Input: part model. Units: mm. Frame: model coordinates. Face numbers are marked on the shaded views. A direction names the side the tool comes from. Coordinates: 2 decimals unless noted, no trailing zeros. Order: outer loops, then holes, each group sorted by start corner. A loop starts at its lowest first (then second) coordinate and runs counter-clockwise, first axis right, second up.
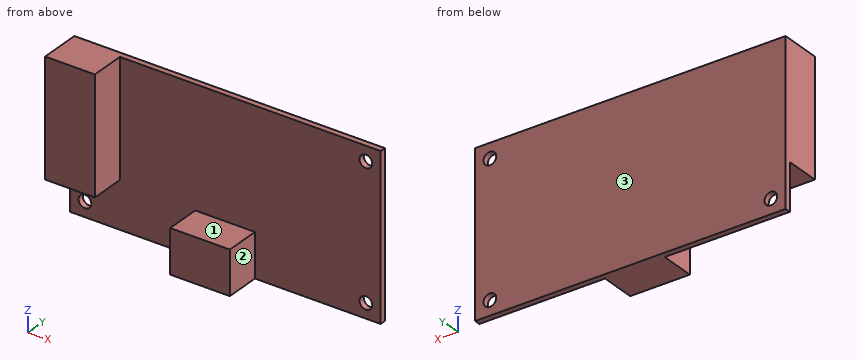
from build123d import *

# Parameters (mm, degrees)
SKETCH1_W           = 53.34
SKETCH1_H           = 27.94
SKETCH1_R           = 1.0922
BOSS_EXTRUDE1_DEPTH = 1
SKETCH2_W           = 8.533603159
SKETCH2_H           = 19.883520928
SKETCH2_W_2         = 10.243705623
SKETCH2_H_2         = 7.528700328
BOSS_EXTRUDE2_DEPTH = 7


with BuildPart() as part:
    # Sketch1 → Boss-Extrude1 (new body)
    with BuildSketch(Plane(origin=(0, 0, 0), x_dir=(1, 0, 0), z_dir=(0, 1, 0))):
        Rectangle(SKETCH1_W, SKETCH1_H)
        with Locations(Location((-24.13, 11.43, 0), (0, 0, 270))):
            Circle(SKETCH1_R, mode=Mode.SUBTRACT)
        with Locations(Location((24.13, 11.43, 0), (0, 0, 270))):
            Circle(SKETCH1_R, mode=Mode.SUBTRACT)
        with Locations(Location((24.13, -11.43, 0), (0, 0, 270))):
            Circle(SKETCH1_R, mode=Mode.SUBTRACT)
    extrude(amount=BOSS_EXTRUDE1_DEPTH)

    # Sketch2 → Boss-Extrude2 (add)
    with BuildSketch(Plane(origin=(0, 1, 0), x_dir=(1, 0, 0), z_dir=(0, 1, 0))):
        with Locations((-22.403198421, -4.028239536)):
            Rectangle(SKETCH2_W, SKETCH2_H)
        with Locations((-0.059974857, 10.205649836)):
            Rectangle(SKETCH2_W_2, SKETCH2_H_2)
    extrude(amount=-BOSS_EXTRUDE2_DEPTH)


solid = part.part
Item 1: Ray query, probe 1 along X at (y, z) = (0.5, -11.43); probe 2 along X at (y, z) = (0.2, 11.43); probe 3 along Z at (x, y) = (5, -0.75). Return the intervals inside material, ascending.
Response values:
probe 1: x = -26.67 to -25.22, -23.04 to 23.04, 25.22 to 26.67
probe 2: x = -26.67 to 23.04, 25.22 to 26.67
probe 3: z = -13.97 to -6.44
Item 2: Cut plane C-C on x = -24.13. Return loops of the section in (y, z), then the cut area to 3 significant figures.
Response values:
outline: (-6, -5.91) - (0, -5.91) - (0, -10.34) - (1, -10.34) - (1, 13.97) - (-6, 13.97) - close; (0, -13.97) - (1, -13.97) - (1, -12.52) - (0, -12.52) - close
area: 145 mm2
Item 3: Cut plane B-B on z = 11.43. Return loops of the section in (x, y).
Response values:
outline: (-26.67, -6) - (-18.14, -6) - (-18.14, 0) - (23.04, 0) - (23.04, 1) - (-26.67, 1) - close; (25.22, 0) - (26.67, 0) - (26.67, 1) - (25.22, 1) - close
Item 4: Cut plane D-D on z = -11.43. Return loops of the section in (x, y), then the cut area to 3 significant figures.
Response values:
outline: (-26.67, 0) - (-25.22, 0) - (-25.22, 1) - (-26.67, 1) - close; (-23.04, 0) - (-5.18, 0) - (-5.18, -6) - (5.06, -6) - (5.06, 0) - (23.04, 0) - (23.04, 1) - (-23.04, 1) - close; (25.22, 0) - (26.67, 0) - (26.67, 1) - (25.22, 1) - close
area: 110 mm2
Item 5: Cut plane A-A on y = -2. Return loops of the section in (x, z).
Response values:
outline: (-26.67, -5.91) - (-18.14, -5.91) - (-18.14, 13.97) - (-26.67, 13.97) - close; (-5.18, -13.97) - (5.06, -13.97) - (5.06, -6.44) - (-5.18, -6.44) - close
Item 6: Access query for the marked faces 1, 2 and 3. Directions: +Z, -Z, +X, -X, +Y, -Y. A direction counts if a zero-diameter tool reaches every point of the face in a straight line with its end or side. Return the directions, or none.
Response values:
face 1: +Z, +X, -X, -Y
face 2: +Z, -Z, +X, -Y
face 3: +Z, -Z, +X, -X, +Y
Item 7: Pin query (flat end, axial travel): pin 1 Ø1.5 at (x, y) = (-16.5, -1.5) entering from +Z; pin 2 Ø3 at (y, z) = (-2.5, 6.5) entering from +X; pin 3 Ø1.5 at (x, z) = (1.5, 1.5) entering from -Y; pin 4 Ø3 at (x, y) = (-1, -3) entering from +Z. Return the tip coordinate at first contact, or that it passes through.
Response values:
pin 1: passes through
pin 2: stops at x = -18.14
pin 3: stops at y = 0
pin 4: stops at z = -6.44
